```python
from build123d import *

# Parameters (mm, degrees)
F0_W     = 82.585936
F0_H     = 97.54353
F1_DEPTH = 25.4
F2_W     = 52.105936
F2_H     = 67.06353
F3_DEPTH = 25.4
F4_R     = 5.08


with BuildPart() as f1:
    # F0 (on Top) → F1 (new body)
    with BuildSketch(Plane.XY):
        with Locations((-11.342247, 4.783943)):
            Rectangle(F0_W, F0_H)
    extrude(amount=F1_DEPTH)

    # F2 (on face) → F3 (cut)
    with BuildSketch(Plane.XY.offset(25.4)):
        with Locations((-11.342247, 4.783943)):
            Rectangle(F2_W, F2_H)
    extrude(amount=-F3_DEPTH, mode=Mode.SUBTRACT)

    # F4
    f4_edges = [f1.edges().sort_by_distance(p)[0] for p in [
        (29.950721, 4.783943, 0),
    ]]
    fillet(f4_edges, radius=F4_R)


solid = f1.part
```
Work out the finished part from the listing and answer in its coordinate system (mm). A direction names the side the tool comes from. Give positions to 0.01 mm unless a question says otherwise; leave off trailing zeros. Write each loop counter-clockwise with the first axis right and the second up, starting at its lowest first coordinate (ties: lowest second). Pieces come first, ordered by that corner, then holes.
(1) The part is cut by section A-A on x = -13. Write down the section's boundary in (y, z).
Final values:
outline: (-43.99, 0) - (-28.75, 0) - (-28.75, 25.4) - (-43.99, 25.4) - close; (38.32, 0) - (53.56, 0) - (53.56, 25.4) - (38.32, 25.4) - close
(2) The part is cut by section C-C on y = -16. Write down the section's boundary in (x, z), plus the area to 3 significant figures.
Final values:
outline: (-52.64, 0) - (-37.4, 0) - (-37.4, 25.4) - (-52.64, 25.4) - close; (14.71, 0) - (24.87, 0) arc R5.08 ccw to (29.95, 5.08) - (29.95, 25.4) - (14.71, 25.4) - close
area: 769 mm2
(3) Which of the six approach directions +Z, -Z, +X, -X, +Y, -Y give full straight-line access (tool end or side, diameter ignored) to faces 4 (the flat face through (16, 5, 25.4)), 5 (the flat face through (-37.395, 4, 13))?
Final values:
face 4: +Z, +X, -X, +Y, -Y
face 5: +Z, -Z
(4) Straight lines are drawn through the part: line 1 (X direction, y = 36, z = 5.5); line 2 (Y direction, x = -6, z = 8); line 3 (X direction, y = 37, z = 2). For each, find the intervals that lie inside material, in ascending order.
Final values:
line 1: x = -52.64 to -37.4, 14.71 to 29.95
line 2: y = -43.99 to -28.75, 38.32 to 53.56
line 3: x = -52.64 to -37.4, 14.71 to 28.91
(5) The mould has two halves that part along X. Classify faces 1 (the cylindrical face through (28.423, 5.467, 1.449)), 2 (the flat face through (-12, -43.988, 13)), 3 (the flat face through (14.711, 4, 13)): pulls with the +X half, pulls with the -X half, needs draft (parallel to the pull), parting line crosses it, or undercut.
Final values:
face 1: pulls with the +X half
face 2: needs draft
face 3: undercut
(6) A flat-ended cylindrical pin translates along its axis: pin 1 Ø12 at (x, y) = (-36.5, -15.5) entering from +Z. Find the tip coordinate at first contact, or state that the pin passes through.
Final values:
pin 1: stops at z = 25.4
(7) The part is cut by section B-B on z = 21. Write down the section's boundary in (x, y).
Final values:
outline: (-52.64, -43.99) - (29.95, -43.99) - (29.95, 53.56) - (-52.64, 53.56) - close; hole (-37.4, -28.75) - (14.71, -28.75) - (14.71, 38.32) - (-37.4, 38.32) - close
